```python
from build123d import *

# Parameters (mm, degrees)
F0_R     = 1.25
F1_DEPTH = 6
F2_R     = 1.25
F3_DEPTH = 64.001


with BuildPart() as f1:
    # F0 (on Top) → F1 (new body)
    with BuildSketch(Plane.XY):
        with BuildLine():
            Line((30.5, -4), (30.5, 5))
            Line((30.5, 5), (-30.5, 5))
            Line((-30.5, 5), (-30.5, -4))
            ThreePointArc((-30.5, -4), (-29.792893, -5.707107), (-31.5, -5))
            Line((-31.5, -5), (-33.5, -5))
            Line((-33.5, -5), (-33.5, -8))
            Line((-33.5, -8), (-28.5, -8))
            ThreePointArc((-28.5, -8), (-26.37868, -7.12132), (-25.5, -5))
            Line((-25.5, -5), (25.5, -5))
            ThreePointArc((25.5, -5), (26.37868, -7.12132), (28.5, -8))
            Line((28.5, -8), (33.5, -8))
            Line((33.5, -8), (33.5, -5))
            Line((33.5, -5), (31.5, -5))
            ThreePointArc((31.5, -5), (29.792893, -5.707107), (30.5, -4))
        make_face()
        with Locations((-18, 0)):
            Circle(F0_R, mode=Mode.SUBTRACT)
        with Locations((18, 0)):
            Circle(F0_R, mode=Mode.SUBTRACT)
    extrude(amount=F1_DEPTH)

    # F2 (on face) → F3 (cut, through all)
    with BuildSketch(Plane.YZ.offset(30.5)):
        with Locations((0, 3)):
            Circle(F2_R)
    extrude(amount=-F3_DEPTH, mode=Mode.SUBTRACT)


solid = f1.part
```
Model file for the job. Use its own axes, mm. A direction names the side the tool comes from. Coordinates: 2 decimals unless noted, no trailing zeros. Order: outer loops, then holes, each group sorted by start corner. A loop starts at its lowest first (then second) coordinate and runs counter-clockwise, first axis right, second up. Notation, with made-up numbers: (-21.75, -16.75) -> (-6.75, -16.75) arc R8 cw to (-6.75, -12.75) -> close; hole circle Ø11 at (32, 16.5). An arc over 180 degrees is marked (long way). Answer as a JSON object with one key per item and string values. Group by question number.
1) Which spindle directions (+Z, -Z, +X, -X, +Y, -Y) get a long thin tool onto all of the face, cutting with end or side? Do faces 4 (the face through (30.5, 1.44, 2.96)), 5 (the face through (-19.25, 0.05, 4.81)), 6 (the face through (0, -5, 3)). Say none if no direction does.
2) Pull direction X, two halves, no side cores. Call faces 1 (the face through (-33.5, -6, 3)), 2 (the face through (-32, -5, 3)), 3 (the face through (-17.328, 1.054, 1.146)): +X half, -X half, draft (parallel to the pull), parting line (faces both ways), or undercut.
3) Flat gauge pins, fed straight in: pin 1 (2 mm diameter, centred on y = -1.5, z = 1, fed in from +X); pin 2 (1.8 mm diameter, centred on y = 2.5, z = 2.5, fed in from -X); pin 3 (1 mm diameter, centred on x = -32.5, z = 4.5, fed in from +Y). Where does each tip first touch, or does it go through?
4) Drill centre lines: L1, parallel to X at y = 0, z = 0.65; L2, parallel to Y at x = 18, z = 2.1; L3, parallel to Z at x = 3.5, y = 0. Where is each one in solid material? Low to high.
5) Cut at B-B, the plane y = 0. Write the cut outline in (x, z), then the cut area to 3 significant figures.
6) Cut at D-D, the plane x = 26.5. Write the cut outline in (y, z), then the cut area to 3 significant figures.
7) Cut at A-A, the plane z = 5.15. Write the cut outline in (x, y), then the cut area to 3 significant figures.
8) Cut at C-C, the plane y = -7. Write the cut outline in (x, z), then the cut area to 3 significant figures.
Check values:
{
 "1": {"face 4": "+Z, -Z, +X, +Y", "face 5": "+Z, -Z", "face 6": "+Z, -Z, -Y"},
 "2": {"face 1": "-X half", "face 2": "draft", "face 3": "undercut"},
 "3": {"pin 1": "stops at x = 30.5", "pin 2": "stops at x = -30.5", "pin 3": "stops at y = -5"},
 "4": {"L1": "x = -30.5 to -19.25, -16.75 to 16.75, 19.25 to 30.5", "L2": "y = -5 to -1.25, 1.25 to 5", "L3": "z = 0 to 1.75, 4.25 to 6"},
 "5": {"outline": "(-30.5, 0) -> (-19.25, 0) -> (-19.25, 1.75) -> (-30.5, 1.75) -> close; (-30.5, 4.25) -> (-19.25, 4.25) -> (-19.25, 6) -> (-30.5, 6) -> close; (-16.75, 0) -> (16.75, 0) -> (16.75, 1.75) -> (-16.75, 1.75) -> close; (-16.75, 4.25) -> (16.75, 4.25) -> (16.75, 6) -> (-16.75, 6) -> close; (19.25, 0) -> (30.5, 0) -> (30.5, 1.75) -> (19.25, 1.75) -> close; (19.25, 4.25) -> (30.5, 4.25) -> (30.5, 6) -> (19.25, 6) -> close", "area": "196 mm²"},
 "6": {"outline": "(-7.24, 0) -> (5, 0) -> (5, 6) -> (-7.24, 6) -> close; hole circle Ø2.5 at (0, 3)", "area": "68.5 mm²"},
 "7": {"outline": "(-33.5, -8) -> (-28.5, -8) arc R3 ccw to (-25.5, -5) -> (25.5, -5) arc R3 ccw to (28.5, -8) -> (33.5, -8) -> (33.5, -5) -> (31.5, -5) arc R1 cw (long way) to (30.5, -4) -> (30.5, 5) -> (-30.5, 5) -> (-30.5, -4) arc R1 cw (long way) to (-31.5, -5) -> (-33.5, -5) -> close; hole circle Ø2.5 at (-18, 0); hole circle Ø2.5 at (18, 0)", "area": "640 mm²"},
 "8": {"outline": "(-33.5, 0) -> (-26.26, 0) -> (-26.26, 6) -> (-33.5, 6) -> close; (26.26, 0) -> (33.5, 0) -> (33.5, 6) -> (26.26, 6) -> close", "area": "86.8 mm²"}
}
